from build123d import *

# Parameters (mm, degrees)
SKETCH1_W           = 8.5
SKETCH1_H           = 10.5
BOSS_EXTRUDE1_DEPTH = 12.5
SKETCH2_W           = 8.5
SKETCH2_H           = 2
CUT_EXTRUDE1_DEPTH  = 8
BOSS_EXTRUDE2_DEPTH = 2
CHAMFER1_SIZE       = 1
SKETCH4_W           = 1.671920984
SKETCH4_H           = 12.5
BOSS_EXTRUDE3_DEPTH = 1


with BuildPart() as part:
    # Sketch1 → Boss-Extrude1 (new body)
    with BuildSketch(Plane.XY):
        Rectangle(SKETCH1_W, SKETCH1_H)
    extrude(amount=BOSS_EXTRUDE1_DEPTH)

    # Sketch2 → Cut-Extrude1 (cut)
    with BuildSketch(Plane.XY.offset(12.5)):
        with Locations((0, -0.25)):
            Rectangle(SKETCH2_W, SKETCH2_H)
    extrude(amount=-CUT_EXTRUDE1_DEPTH, mode=Mode.SUBTRACT)

    # Sketch3 → Boss-Extrude2 (add)
    # profile 1 of 2: a face of its own
    with BuildSketch(Plane.XZ.offset(5.25)):
        with BuildLine():
            Line((4.25, 0), (8, 0))
            ThreePointArc((8, 0), (9.414213562, 0.585786438), (10, 2))
            Line((10, 2), (10, 5))
            ThreePointArc((10, 5), (9.414213562, 6.414213562), (8, 7))
            Line((8, 7), (4.25, 7))
            Line((4.25, 7), (4.25, 0))
        make_face()
        with BuildLine():
            Line((6, 2.5), (6, 3.5))
            ThreePointArc((6, 3.5), (7.5, 5), (9, 3.5))
            Line((9, 3.5), (9, 2.5))
            ThreePointArc((9, 2.5), (7.5, 1), (6, 2.5))
        make_face(mode=Mode.SUBTRACT)
    # profile 2 of 2: a face of its own
    with BuildSketch(Plane.XZ.offset(5.25)):
        with BuildLine():
            Line((-10, 2), (-10, 5))
            ThreePointArc((-10, 5), (-9.414213562, 6.414213562), (-8, 7))
            Line((-8, 7), (-4.25, 7))
            Line((-4.25, 7), (-4.25, 0))
            Line((-4.25, 0), (-8, 0))
            ThreePointArc((-8, 0), (-9.414213562, 0.585786438), (-10, 2))
        make_face()
        with BuildLine():
            Line((-6, 2.5), (-6, 3.5))
            ThreePointArc((-6, 3.5), (-7.5, 5), (-9, 3.5))
            Line((-9, 3.5), (-9, 2.5))
            ThreePointArc((-9, 2.5), (-7.5, 1), (-6, 2.5))
        make_face(mode=Mode.SUBTRACT)
    extrude(amount=-BOSS_EXTRUDE2_DEPTH)

    # Chamfer1
    chamfer1_edges = [part.edges().sort_by_distance(p)[0] for p in [
        (-4.25, 3, 12.5),
        (4.25, 3, 12.5),
        (-4.25, -3.25, 12.5),
        (4.25, -3.25, 12.5),
    ]]
    chamfer(chamfer1_edges, length=CHAMFER1_SIZE)

    # Sketch4 → Boss-Extrude3 (add)
    with BuildSketch(Plane.XZ.offset(5.25)):
        with Locations((0, 6.25)):
            Rectangle(SKETCH4_W, SKETCH4_H)
    extrude(amount=BOSS_EXTRUDE3_DEPTH)


solid = part.part
CAD build for the part. Positions are in the model's coordinates, mm. A direction names the side the tool comes from. Round coordinates to 2 decimals unless told otherwise and drop trailing zeros. Order: outer loops, then holes, each group sorted by start corner. A loop starts at its lowest first (then second) coordinate and runs counter-clockwise, first axis right, second up. Notation, with made-up numbers: (23, 48) -> (56, 48) arc R24 cw to (56, 75) -> close; hole circle Ø6 at (38, -23). An arc over 180 degrees is marked (long way). Write item = value, one per line. Start each with the question number.
(1) Cut at D-D, the plane x = -2.25. List the corners of the cut face in (y, z), then the cut area to 3 significant figures.
(2) Pin check, flat tips, straight feed: P1, Ø1.1, axis at y = -6, z = 9.5, coming from the -X side; P2, Ø3, axis at x = 4, z = 7.5, coming from the -Y side; P3, Ø6, axis at x = 1.5, z = 3.5, coming from the -Y side; P4, Ø1, axis at x = 6, y = -4, coming from the +Z side. Stop position of each tip, or through.
(3) Cut at A-A, the plane y = -5. List the corners of the cut face in (x, z), then the cut area to 3 significant figures.
(4) Pull direction X, two halves, no side cores. Call faces 6 (the flat face through (-0.836, -6, 6)), 7 (the flat face through (0, -3, 12.5)), 8 (the cylindrical face through (-7.5, -4.3, 1)): released by +X, released by -X, zero draft, split by the parting line, or undercut.
(5) Cut at B-B, the plane x = -7.5. List the corners of the cut face in (y, z).
(6) Cut at C-C, the plane z = 6. List the corners of the cut face in (x, y).
(7) Probe line 1 (Y direction, x = 2.25, z = 8); line 2 (Y direction, x = -0.5, z = 11.25); line 3 (Z direction, x = 7.5, y = -3.75). List the from-to ranges inside material, lowest first. Write a range as [from, to].
(8) Which spindle directions (+Z, -Z, +X, -X, +Y, -Y) get a long thin tool onto all of the face, cutting with end or side? Do faces 1 (the flat face through (5.8, -3.25, 3.5)), 2 (the flat face through (-9, -4, 3)), 3 (the flat face through (4, -5.25, 5)), 4 (the flat face through (0, -1.25, 9)), 5 (the flat face through (-5.8, -3.25, 3.5)). Say none if no direction does.
Model answer:
q1.outline = (-5.25, 0) -> (5.25, 0) -> (5.25, 12.5) -> (0.75, 12.5) -> (0.75, 4.5) -> (-1.25, 4.5) -> (-1.25, 12.5) -> (-5.25, 12.5) -> close
q1.area = 115 mm2
q2.P1 = -0.84
q2.P2 = -5.25
q2.P3 = -6.25
q2.P4 = 7
q3.outline = (-10, 2) arc R2 ccw to (-8, 0) -> (8, 0) arc R2 ccw to (10, 2) -> (10, 5) arc R2 ccw to (8, 7) -> (4.25, 7) -> (4.25, 11.5) -> (3.25, 12.5) -> (-3.25, 12.5) -> (-4.25, 11.5) -> (-4.25, 7) -> (-8, 7) arc R2 ccw to (-10, 5) -> close; hole (-9, 2.5) arc R1.5 ccw to (-6, 2.5) -> (-6, 3.5) arc R1.5 ccw to (-9, 3.5) -> close; hole (6, 2.5) arc R1.5 ccw to (9, 2.5) -> (9, 3.5) arc R1.5 ccw to (6, 3.5) -> close
q3.area = 162 mm2
q4.face_6 = released by -X
q4.face_7 = zero draft
q4.face_8 = undercut
q5.outline = (-5.25, 0) -> (-3.25, 0) -> (-3.25, 1) -> (-5.25, 1) -> close; (-5.25, 5) -> (-3.25, 5) -> (-3.25, 7) -> (-5.25, 7) -> close
q6.outline = (-9.73, -5.25) -> (-0.84, -5.25) -> (-0.84, -6.25) -> (0.84, -6.25) -> (0.84, -5.25) -> (9.73, -5.25) -> (9.73, -3.25) -> (4.25, -3.25) -> (4.25, -1.25) -> (-4.25, -1.25) -> (-4.25, -3.25) -> (-9.73, -3.25) -> close; (-4.25, 0.75) -> (4.25, 0.75) -> (4.25, 5.25) -> (-4.25, 5.25) -> close
q7.line_1 = [-5.25, -1.25], [0.75, 5.25]
q7.line_2 = [-6.25, -1.25], [0.75, 5.25]
q7.line_3 = [0, 1], [5, 7]
q8.face_1 = +Z, -Z, +X, +Y
q8.face_2 = +Y, -Y
q8.face_3 = +Z, -Z, +X, -Y
q8.face_4 = +Z, +X, -X
q8.face_5 = +Z, -Z, -X, +Y
